Here's how the part is built. I have some questions about the finished solid (model axes, mm). A direction names the side the tool comes from. Coordinates: 2 decimals unless noted, no trailing zeros. Write each loop counter-clockwise with the first axis right and the second up, starting at its lowest first coordinate (ties: lowest second). Pieces come first, ordered by that corner, then holes. Notation, with made-up numbers: (-21, 62.25) -> (-4, 62.25) arc R25 ccw to (-4, 79.25) -> close; hole circle Ø8 at (75, 48). An arc over 180 degrees is marked (long way). Answer in a Markdown table with one row per item. Add a question column.
Autodesk Inventor part; units mm, degrees
ref_plane "Work Plane1" through (5, 0, 0) normal (0, 0, 1) x (1, 0, 0)
ref_plane "YZ Plane" through (0, 0, 0) normal (1, 0, 0) x (0, 1, 0)
ref_plane "XZ Plane" through (0, 0, 0) normal (0, 1, 0) x (-1, 0, 0)
sketch "Эскиз1" plane through (0, 0, 0) normal (0, 0, 1) x (1, 0, 0)
  line L0 (0, 0) -> (3.6667, 0)
  line L1 (10, 2.3094) -> (10, 4)
  line L2 (10, 4) -> (0, 4)
  line L3 (10, 2.3094) -> (5, 2.3094)
  line L4 (5, 2.3094) -> (3.6667, 0)
  line L5 (0, -0.8) -> (0, 4.8)
  line L6 (0, 4) -> (0, 0)
  dimension "d0" = 5
  dimension "d1" = 60
  dimension "d2" = 8
  dimension "d3" = 4.6188
  dimension "d5" = 10
revolve "Базовый элемент" add sketch "Эскиз1" angle 360 about axis through (0, 0, 0) along (1, 0, 0)
sketch "Эскиз2" plane through (10, 0, 0) normal (1, 0, 0) x (0, 1, 0)
  circle A0 centre (0, 0) radius 2.3094
  line L0 (-1.1547, 2) -> (1.1547, 2)
  line L1 (1.1547, 2) -> (2.3094, 0)
  line L2 (2.3094, 0) -> (1.1547, -2)
  line L3 (1.1547, -2) -> (-1.1547, -2)
  line L4 (-1.1547, -2) -> (-2.3094, 0)
  line L5 (-2.3094, 0) -> (-1.1547, 2)
  point P0 (0, 0)
  point P1 (0, 0)
extrude "Паз" add sketch "Эскиз2" against normal up to next contours L1 A0 | A0 L2 | L0 A0 | A0 L3 | L5 A0 | A0 L4
thread "Резьба"
chamfer "Фаска1" distance 1.7321 angle 60 1 edges at (0, -4, 0) measured on face at (6.6667, 3.987, -0.3219)
chamfer "Фаска2" distance 0.7668 angle 60 1 edges at (10, -4, 0) measured on face at (7.244, 3.9482, -0.6416)
ref_plane "Work Plane1" through (5, 0, 0) normal (0, 0, 1) x (1, 0, 0)
equation "\"d0\" = INTI"
equation "\"d2\" = NND"
equation "\"d3\" = 1.1547 * SW"
equation "\"d5\" = NLG"
equation "\"d12\" = NLG"
equation "\"d9\" = FAWI"
equation "\"d10\" = -0.5 * GD1 + 0.5 * NND"
equation "\"d11\" = FAWI"
equation "\"d35\" = -0.5 * GD1 + 0.5 * NND"
equation "\"NND\" = 8"
equation "\"NLG\" = 10"
equation "\"INTI\" = 5"
equation "\"FAWI\" = 60deg"
equation "\"SW\" = 4"
equation "\"GD1\" = THREADDIA - 1.2269 * PTC"
equation "\"FAWI1\" = 45deg"
equation "\"SPD\" = 2"
equation "\"GUL\" = 0.61345 * PTC"
equation "\"TOA\" = 30deg"
equation "\"THREADDIA\" = 8"
equation "\"PTC\" = 1.25"
equation "\"GAL\" = 0.61345 * PTC"
equation "\"E0\" = 1.155 * SW"
properties part number "AS 1421 - M8x10 конический" material "Сталь, мягкая"
Q1. If we mould it in two halves opening along Z, with no side actions, what happens to faces 1 (the cylindrical face through (5.43, -0.867, 3.905)), 2 (the flat face through (10, -2, 1)), 3 (the flat face through (7.45, -1.74, 0.99))? For each: pulls with the +Z half, pulls with the -Z half, needs draft (parallel to the pull), parting line crosses it, or undercut.
Q2. I'm going to push flat-ended pins straight in: P1, Ø2, axis at x = 6.5, y = -2.5, coming from the +Z side; P2, Ø2, axis at x = 9, z = -2, coming from the -Y side; P3, Ø0.7, axis at x = 6, y = -0.5, coming from the +Z side. Where does each tip first touch, or does it pass through?
Q3. I need wall thicknesses on line 1 (Z direction, x = 7.25, y = -0.5); line 2 (Y direction, x = 8, z = 0.25); line 3 (Z direction, x = 5.25, y = -1). Which ranges of each line are inside material? Lowest first, please. Write a range as [from, to].
Q4. Imagine slicing it at A-A on x = 5.5. Please give me the cut outline in (y, z).
Q5. For faces 4 (the flat face through (7.447, 1.724, 1.014)), 5 (the flat face through (0, 0, 0)), which set-ups out of +Z, -Z, +X, -X, +Y, -Y let a thin tool reach every point of the face, with its end or its side?
Q6. Imagine slicing it at B-B on x = 2.75. Please give me the cut outline in (y, z), plus the area to 3 significant figures.
Result sheet:
| question | item | result |
|---|---|---|
| 1 | face 1 | parting line crosses it |
| 1 | face 2 | needs draft |
| 1 | face 3 | undercut |
| 2 | P1 | stops at z = 3.71 |
| 2 | P2 | stops at y = -3.87 |
| 2 | P3 | stops at z = 4 |
| 3 | line 1 | z = [-3.97, -2], [2, 3.97] |
| 3 | line 2 | y = [-3.99, -2.17], [2.17, 3.99] |
| 3 | line 3 | z = [-3.87, -2], [2, 3.87] |
| 4 | outline | circle Ø8 at (0, 0); hole (-2.31, 0) -> (-1.15, -2) -> (1.15, -2) -> (2.31, 0) -> (1.15, 2) -> (-1.15, 2) -> close |
| 5 | face 4 | +X |
| 5 | face 5 | +Z, -Z, -X, +Y, -Y |
| 6 | outline | circle Ø8 at (0, 0) |
| 6 | area | 50.3 mm^2 |
